Check sheet for the drawn part. Datum: minimum x, y, z corner. Units: mm. A direction names the side the tool comes from. Give positions to 0.01 mm unless a question says otherwise; leave off trailing zeros. Order: outer loops, then holes, each group sorted by start corner. A loop starts at its lowest first (then second) coordinate and runs counter-clockwise, first axis right, second up.
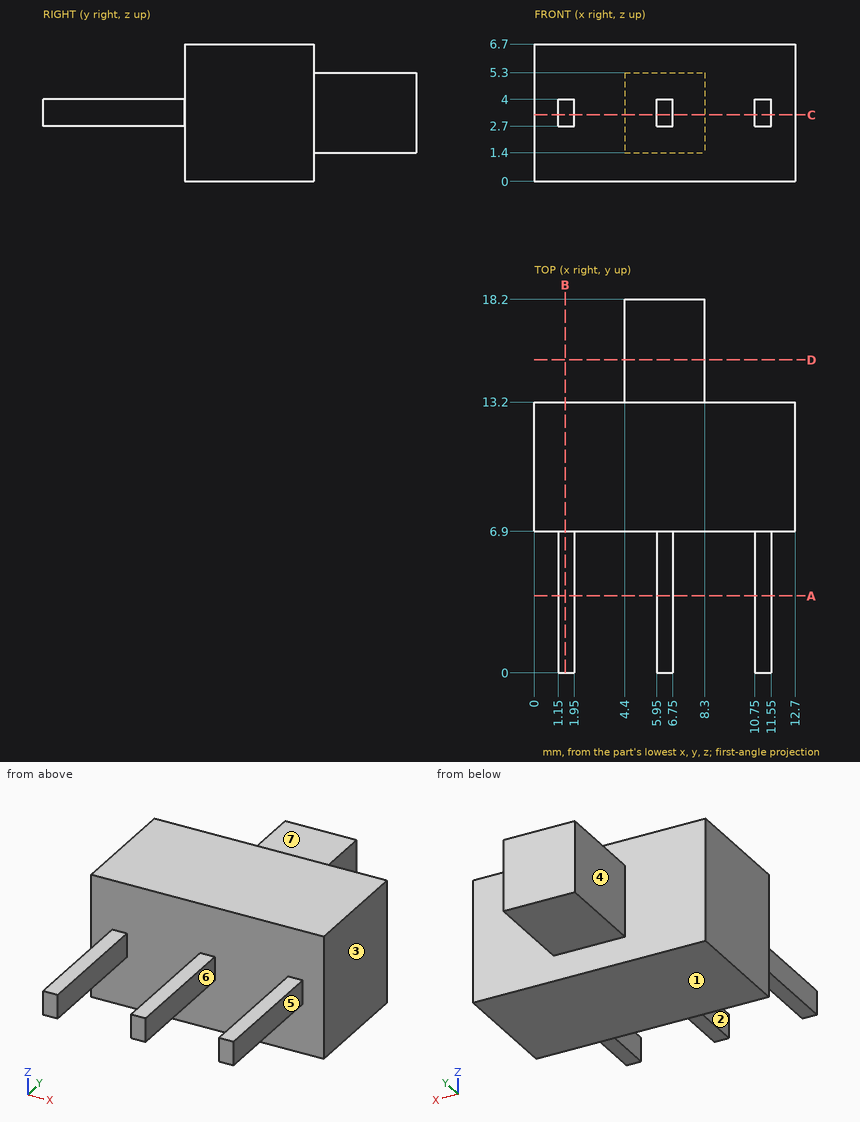
(1) Section check B-B, the plane x = 1.5. Enter the section's corners in (y, z), then the cut area to 3 significant figures.
Solved:
outline: (0, 2.7) - (6.9, 2.7) - (6.9, 0) - (13.2, 0) - (13.2, 6.7) - (6.9, 6.7) - (6.9, 4) - (0, 4) - close
area: 51.2 mm2
(2) Section check A-A, the plane y = 3.75. Enter the section's corners in (x, z), then the cut area to 3 significant figures.
Solved:
outline: (1.15, 2.7) - (1.95, 2.7) - (1.95, 4) - (1.15, 4) - close; (5.95, 2.7) - (6.75, 2.7) - (6.75, 4) - (5.95, 4) - close; (10.75, 2.7) - (11.55, 2.7) - (11.55, 4) - (10.75, 4) - close
area: 3.12 mm2
(3) Set-up check for the marked faces 4, 5, 6 and 7: record each of +Z, -Z, +X, -X, +Y, -Y from which the full face is reachable in a straight line by a thin tool's end or side.
Solved:
face 4: +Z, -Z, -X, +Y
face 5: +Z, -Z, +X, -Y
face 6: +Z, -Z, -Y
face 7: +Z, +X, -X, +Y
(4) Scan lines: line 1 (X direction, y = 5, z = 3.25); line 2 (X direction, y = 13.25, z = 2.5); line 3 (Y direction, x = 4.25, z = 1.5). Record each from-to range of solid material in increasing order.
Solved:
line 1: x = 1.15 to 1.95, 5.95 to 6.75, 10.75 to 11.55
line 2: x = 4.4 to 8.3
line 3: y = 6.9 to 13.2
(5) Section check D-D, the plane y = 15.25. Enter the section's corners in (x, z).
Solved:
outline: (4.4, 1.4) - (8.3, 1.4) - (8.3, 5.3) - (4.4, 5.3) - close
(6) Go/stop test with flat-tipped pins: pin 1 (4.5 mm diameter, centred on x = 6.5, y = 16.5, fed in from +Z); pin 2 (1 mm diameter, centred on y = 3, z = 3, fed in from +X); pin 3 (0.6 mm diameter, centred on x = 6, y = 4, fed in from -Z). Record where each tip stops, or that it passes through.
Solved:
pin 1: stops at z = 5.3
pin 2: stops at x = 11.55
pin 3: stops at z = 2.7
(7) Release check for a two-part mould opening along X. For the marked faces 1, 2 and 3 record: pulls with the +X half, pulls with the -X half, needs draft (parallel to the pull), parting line crosses it, or undercut.
Solved:
face 1: needs draft
face 2: undercut
face 3: pulls with the +X half
(8) Section check C-C, the plane z = 3.25. Enter the section's corners in (x, y), then the cut area to 3 significant figures.
Solved:
outline: (0, 6.9) - (1.15, 6.9) - (1.15, 0) - (1.95, 0) - (1.95, 6.9) - (5.95, 6.9) - (5.95, 0) - (6.75, 0) - (6.75, 6.9) - (10.75, 6.9) - (10.75, 0) - (11.55, 0) - (11.55, 6.9) - (12.7, 6.9) - (12.7, 13.2) - (8.3, 13.2) - (8.3, 18.2) - (4.4, 18.2) - (4.4, 13.2) - (0, 13.2) - close
area: 116 mm2
